Source: CAD feature listing. Evaluate the final solid. Frame: model axes, mm. A direction names the side the tool comes from. Give positions to 0.01 mm unless a question says otherwise; leave off trailing zeros. Order: outer loops, then holes, each group sorted by start corner. A loop starts at its lowest first (then second) coordinate and runs counter-clockwise, first axis right, second up. Notation, with made-up numbers: (13, 13) - (29, 13) arc R28 cw to (29, 52) - close; hole circle Ø2 at (3.5, 13.25). An arc over 180 degrees is marked (long way). Answer as CSV lines item,"result".
```python
from build123d import *

# Parameters (mm, degrees)
SKETCH2_R           = 20
BOSS_EXTRUDE2_DEPTH = 120
SKETCH2_3_R         = 20
BOSS_EXTRUDE3_DEPTH = 120
CUT_EXTRUDE1_DEPTH  = 95
CUT_EXTRUDE2_DEPTH  = 26
CUT_EXTRUDE3_DEPTH  = 28
CUT_EXTRUDE4_DEPTH  = 3


with BuildPart() as part:
    # Sketch2 → Boss-Extrude2 (new body)
    with BuildSketch(Plane.XY):
        Circle(SKETCH2_R)
    extrude(amount=BOSS_EXTRUDE2_DEPTH)

    # Sketch2_3 → Boss-Extrude3 (add)
    with BuildSketch(Plane.XY):
        Circle(SKETCH2_3_R)
    extrude(amount=BOSS_EXTRUDE3_DEPTH)

    # Sketch4 → Cut-Extrude1 (cut)
    with BuildSketch(Plane.XY.offset(120)):
        with BuildLine():
            Line((-20, 0), (20, 0))
            ThreePointArc((20, 0), (0, 20), (-20, 0))
        make_face()
    extrude(amount=-CUT_EXTRUDE1_DEPTH, mode=Mode.SUBTRACT)

    # Sketch5 → Cut-Extrude2 (cut, through all)
    with BuildSketch(Plane.XY.offset(25)):
        with BuildLine():
            ThreePointArc((16, 0), (0, 16), (-16, 0))
            Line((-16, 0), (16, 0))
        make_face()
    extrude(amount=-CUT_EXTRUDE2_DEPTH, mode=Mode.SUBTRACT)

    # Sketch6 → Cut-Extrude3 (cut)
    with BuildSketch(Plane.XY.offset(120)):
        with BuildLine():
            Line((-10, 0), (-16, 0))
            ThreePointArc((-16, 0), (0, -16), (16, 0))
            Line((16, 0), (10, 0))
            ThreePointArc((10, 0), (0, -10), (-10, 0))
        make_face()
    extrude(amount=-CUT_EXTRUDE3_DEPTH, mode=Mode.SUBTRACT)

    # Sketch7 → Cut-Extrude4 (cut)
    with BuildSketch(Plane(origin=(0, 0, 0), x_dir=(1, 0, 0), z_dir=(0, 1, 0))):
        with BuildLine():
            Line((0, -85), (0, -30))
            ThreePointArc((0, -30), (-3.535533906, -31.464466094), (-5, -35))
            Line((-5, -35), (-5, -80))
            ThreePointArc((-5, -80), (-3.535533906, -83.535533906), (0, -85))
        make_face()
        with BuildLine():
            ThreePointArc((5, -35), (3.535533906, -31.464466094), (0, -30))
            Line((0, -30), (0, -85))
            ThreePointArc((0, -85), (3.535533906, -83.535533906), (5, -80))
            Line((5, -80), (5, -35))
        make_face()
    extrude(amount=-CUT_EXTRUDE4_DEPTH, mode=Mode.SUBTRACT)


solid = part.part
```
(1) Cut plane B-B (x = 2.5). Return loops of the section in (y, z), then the cut area to 3 significant figures.
Completed:
outline,"(-19.84, 0) - (0, 0) - (0, 30.67) - (-3, 30.67) - (-3, 84.33) - (0, 84.33) - (0, 120) - (-9.68, 120) - (-9.68, 92) - (-15.8, 92) - (-15.8, 120) - (-19.84, 120) - close; (15.8, 0) - (19.84, 0) - (19.84, 25) - (15.8, 25) - close"
area,"2,150 mm²"
(2) Ray query, line 1 (X direction, y = -0.5, z = 52.5); line 2 (Z direction, x = -6, y = 18.5); line 3 (Y direction, x = -12, z = 84). Return the intervals inside material, ascending. Write a range as from..to.
Completed:
line 1,"-19.99..-5, 5..19.99"
line 2,"0..25"
line 3,"-16..0"
(3) Cut plane D-D (z = 40). Return loops of the section in (x, y), then the cut area to 3 significant figures.
Completed:
outline,"(-20, 0) arc R20 ccw to (20, 0) - (5, 0) - (5, -3) - (-5, -3) - (-5, 0) - close"
area,"598 mm²"
(4) Access query for faces 1 (the flat face through (5, -1, 58)), 2 (the cylindrical face through (0, 16, 13)), 3 (the flat face through (3, 16, 25)), 4 (the cylindrical face through (0, -16, 106)). Directions: +Z, -Z, +X, -X, +Y, -Y. A direction counts if a zero-diameter tool reaches every point of the face in a straight line with its end or side. Return the directions, or none.
Completed:
face 1,"+Y"
face 2,"+Z, -Z"
face 3,"+Z, +X, -X, +Y"
face 4,"+Z"
(5) Cut plane A-A (z = 111). Return loops of the section in (x, y), then the cut area to 3 significant figures.
Completed:
outline,"(-20, 0) arc R20 ccw to (20, 0) - (16, 0) arc R16 cw to (-16, 0) - close; (-10, 0) arc R10 ccw to (10, 0) - close"
area,"383 mm²"
(6) Mould query, pull axis Y, two halves, no side actions, for faces 5 (the flat face through (0, -3, 57)), 6 (the flat face through (-5, -1, 57)), 7 (the cylindrical face through (0, -10, 106)). Classes: released by +Y, released by -Y, zero draft, split by the parting line, or undercut.
Completed:
face 5,"released by +Y"
face 6,"zero draft"
face 7,"undercut"
(7) Contact query for flat-ended pins moving along their axis: pin 1 (6 mm diameter, centred on x = -1.5, z = 43.5, fed in from +Y); pin 2 (1 mm diameter, centred on x = -0.5, z = 97.5, fed in from +Y); pin 3 (3 mm diameter, centred on y = -3.5, z = 17.5, fed in from +X). Output: stop coordinate, or through.
Completed:
pin 1,"y = -3"
pin 2,"y = 0"
pin 3,"x = 19.9"
(8) Cut plane C-C (z = 8.5). Return loops of the section in (x, y), then the cut area to 3 significant figures.
Completed:
outline,"circle Ø40 at (0, 0); hole (-16, 0) - (16, 0) arc R16 ccw to start"
area,"855 mm²"
